Input: part model. Units: mm. Frame: model coordinates. Face numbers are marked on the shaded views. A direction names the side the tool comes from. Round coordinates to 2 decimals unless told otherwise and drop trailing zeros. Loops run counter-clockwise (first coordinate to the right, second up) from the corner with the lowest first, then second, coordinate; pieces in that order, holes last. Notation, with made-up numbers: (-29, -17) - (-14, -17) arc R12 cw to (-14, 5) - close; hole circle Ø11 at (47, 87). An arc over 180 degrees is marked (long way). Write each question's results on one line, items separated by ' | '.
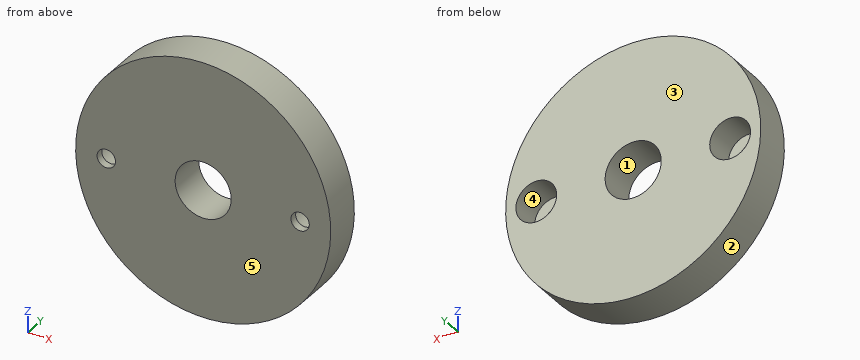
from build123d import *

# Parameters (mm, degrees)
SKETCH1_R           = 25
SKETCH1_R_2         = 1.8
SKETCH1_R_3         = 5.5
BOSS_EXTRUDE1_DEPTH = 7.5
SKETCH2_R           = 4
CUT_EXTRUDE1_DEPTH  = 6


with BuildPart() as part:
    # Sketch1 → Boss-Extrude1 (new body)
    with BuildSketch(Plane(origin=(0, 0, 0), x_dir=(1, 0, 0), z_dir=(0, 1, 0))):
        with Locations(Location((0, 0, 0), (0, 0, 270))):
            Circle(SKETCH1_R)
        with Locations(Location((-19, 0, 0), (0, 0, 270))):
            Circle(SKETCH1_R_2, mode=Mode.SUBTRACT)
        with Locations(Location((19, 0, 0), (0, 0, 90))):
            Circle(SKETCH1_R_2, mode=Mode.SUBTRACT)
        with Locations(Location((0, 0, 0), (0, 0, 270))):
            Circle(SKETCH1_R_3, mode=Mode.SUBTRACT)
    extrude(amount=BOSS_EXTRUDE1_DEPTH)

    # Sketch2 → Cut-Extrude1 (cut)
    with BuildSketch(Plane(origin=(0, 7.5, 0), x_dir=(1, 0, 0), z_dir=(0, 1, 0))):
        with Locations(Location((-19, 0, 0), (0, 0, 270))):
            Circle(SKETCH2_R)
        with Locations(Location((19, 0, 0), (0, 0, 270))):
            Circle(SKETCH2_R)
    extrude(amount=-CUT_EXTRUDE1_DEPTH, mode=Mode.SUBTRACT)


solid = part.part
1. Line query: line 1 (X direction, y = 2.75, z = 0); line 2 (X direction, y = 0.95, z = 0); line 3 (Z direction, x = -19, y = 0.5). Output: solid intervals per line, ascending. Write a range as [from, to].
Answer:
line 1: [-25, -23], [-15, -5.5], [5.5, 15], [23, 25] | line 2: [-25, -20.8], [-17.2, -5.5], [5.5, 17.2], [20.8, 25] | line 3: [-16.25, -1.8], [1.8, 16.25]
2. Mould query, pull axis X, two halves, no side actions, for the marked faces 1, 2 and 3. Classes: pulls with the +X half, pulls with the -X half, needs draft (parallel to the pull), parting line crosses it, or undercut.
Answer:
face 1: undercut | face 2: parting line crosses it | face 3: needs draft
3. Section query A-A, the plane z = 0. Output: boundary loops of the cut face in (x, y), plus the area to 3 significant figures.
Answer:
outline: (-25, 0) - (-20.8, 0) - (-20.8, 1.5) - (-23, 1.5) - (-23, 7.5) - (-25, 7.5) - close; (-17.2, 0) - (-5.5, 0) - (-5.5, 7.5) - (-15, 7.5) - (-15, 1.5) - (-17.2, 1.5) - close; (5.5, 0) - (17.2, 0) - (17.2, 1.5) - (15, 1.5) - (15, 7.5) - (5.5, 7.5) - close; (20.8, 0) - (25, 0) - (25, 7.5) - (23, 7.5) - (23, 1.5) - (20.8, 1.5) - close | area: 186 mm^2
4. Section query D-D, the plane x = 19. Output: boundary loops of the cut face in (y, z), plus the area to 3 significant figures.
Answer:
outline: (0, -16.25) - (7.5, -16.25) - (7.5, -4) - (1.5, -4) - (1.5, -1.8) - (0, -1.8) - close; (0, 1.8) - (1.5, 1.8) - (1.5, 4) - (7.5, 4) - (7.5, 16.25) - (0, 16.25) - close | area: 190 mm^2
5. Set-up query: the marked faces 4 and 5. Return all of +Z, -Z, +X, -X, +Y, -Y with unobstructed straight access to the full face (end or side cutting, diameter ignored); none if empty.
Answer:
face 4: +Y | face 5: +Z, -Z, +X, -X, -Y
6. Section query B-B, the plane x = 0. Output: boundary loops of the cut face in (y, z).
Answer:
outline: (0, -25) - (7.5, -25) - (7.5, -5.5) - (0, -5.5) - close; (0, 5.5) - (7.5, 5.5) - (7.5, 25) - (0, 25) - close
7. Contact query for flat-ended pins moving along their axis: pin 1 (1.5 mm diameter, centred on x = 0.5, z = 11, fed in from -Y); pin 2 (3 mm diameter, centred on x = -19, z = 0, fed in from -Y). Output: stop coordinate, or through.
Answer:
pin 1: y = 0 | pin 2: through
8. Section query C-C, the plane y = 3. Output: boundary loops of the cut face in (x, z), plus the area to 3 significant figures.
Answer:
outline: circle Ø50 at (0, 0); hole circle Ø8 at (-19, 0); hole circle Ø11 at (0, 0); hole circle Ø8 at (19, 0) | area: 1,770 mm^2
